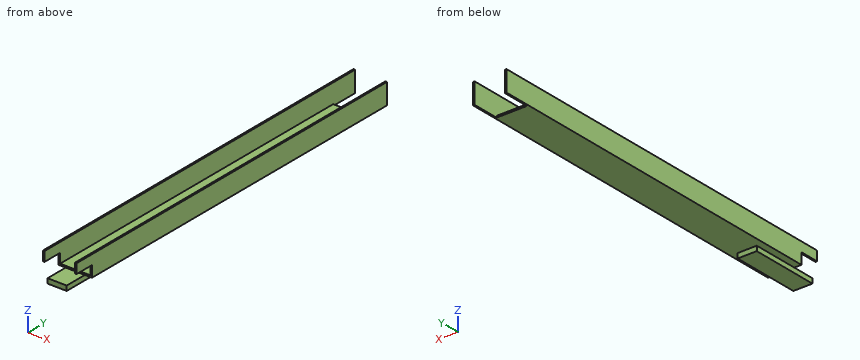
```python
from build123d import *

# Parameters (mm, degrees)
BOSS_EXTRUDE1_DEPTH = 240
SKETCH3_W           = 19
SKETCH3_H           = 1
CUT_EXTRUDE1_DEPTH  = 17
SKETCH4_W           = 19
SKETCH4_H           = 1
CUT_EXTRUDE2_DEPTH  = 11
SKETCH5_W           = 12
SKETCH5_H           = 30
BOSS_EXTRUDE2_DEPTH = 3
SKETCH6_W           = 12
SKETCH6_H           = 3
BOSS_EXTRUDE3_DEPTH = 13
SKETCH7_W           = 7
SKETCH7_H           = 12
CUT_EXTRUDE3_DEPTH  = 30


with BuildPart() as part:
    # Sketch2 → Boss-Extrude1 (new body)
    with BuildSketch(Plane(origin=(0, 0, 0), x_dir=(1, 0, 0), z_dir=(0, 1, 0))):
        Polygon((-10.5, -6.5), (-10.5, 6.5), (10.5, 6.5), (10.5, -6.5), (9.5, -6.5), (9.5, 5.5), (-9.5, 5.5), (-9.5, -6.5), align=None)
    extrude(amount=BOSS_EXTRUDE1_DEPTH)

    # Sketch3 → Cut-Extrude1 (cut)
    with BuildSketch(Plane(origin=(0, 240, 0), x_dir=(1, 0, 0), z_dir=(0, 1, 0))):
        with Locations((0, 6)):
            Rectangle(SKETCH3_W, SKETCH3_H)
    extrude(amount=-CUT_EXTRUDE1_DEPTH, mode=Mode.SUBTRACT)

    # Sketch4 → Cut-Extrude2 (cut)
    with BuildSketch(Plane.XZ):
        with Locations((0, -6)):
            Rectangle(SKETCH4_W, SKETCH4_H)
    extrude(amount=-CUT_EXTRUDE2_DEPTH, mode=Mode.SUBTRACT)

    # Sketch5 → Boss-Extrude2 (add)
    with BuildSketch(Plane(origin=(0, 0, -6.5), x_dir=(-1, 0, 0), z_dir=(0, 0, -1))):
        with Locations((0, 26)):
            Rectangle(SKETCH5_W, SKETCH5_H)
    extrude(amount=BOSS_EXTRUDE2_DEPTH)

    # Sketch6 → Boss-Extrude3 (add)
    with BuildSketch(Plane.XZ.offset(-11)):
        with Locations((0, -8)):
            Rectangle(SKETCH6_W, SKETCH6_H)
    extrude(amount=BOSS_EXTRUDE3_DEPTH)

    # Sketch7 → Cut-Extrude3 (cut)
    with BuildSketch(Plane(origin=(10.5, 0, 0), x_dir=(0, 0, -1), z_dir=(1, 0, 0))):
        with Locations((3, 6)):
            Rectangle(SKETCH7_W, SKETCH7_H)
    extrude(amount=-CUT_EXTRUDE3_DEPTH, mode=Mode.SUBTRACT)


solid = part.part
```
Can you work these out from the model? Positions are in its coordinate system, mm. Coordinates: 2 decimals unless noted, no trailing zeros. Loops run counter-clockwise (first coordinate to the right, second up) from the corner with the lowest first, then second, coordinate; pieces in that order, holes last. Notation, with made-up numbers: M 58,1 L 94,1 A17 ccw 94,20 Z; hole C -35.5,79.25 d4. An arc over 180 degrees is marked long. Put each result on its own line as item: value. Start each with the question number.
(1) Imagine slicing it at D-D on y = 103.5. List the corners of the cut face in (x, z) for me.
(2) Will these pins go through, and if not, where does the flat tip stop? pin 1 Ø0.8 at (x, y) = (-10, 7.5) entering from -Z; pin 2 Ø1 at (x, y) = (8, 188) entering from -Z; pin 3 Ø0.9 at (y, z) = (22, -7.5) entering from -X.
(3) I need wall thicknesses on probe 1 along X at (y, z) = (49, 1.75); probe 2 along Y at (x, z) = (-5.75, -6.25); probe 3 along Z at (x, y) = (-1.25, 8). Which ranges of each line are inside material? Lowest first, please.
(4) Imagine slicing it at B-B on y = 37.5. List the corners of the cut face in (x, z) for me.
(5) Imagine slicing it at A-A on z = -3.5. List the corners of the cut face in (x, y) for me, and give its area (3 significant figures).
(6) Imagine slicing it at C-C on x = -2.75. List the corners of the cut face in (y, z) for me, and give its area (3 significant figures).
Worked answers:
1. outline: M -10.5,-6.5 L 10.5,-6.5 L 10.5,6.5 L 9.5,6.5 L 9.5,-5.5 L -9.5,-5.5 L -9.5,6.5 L -10.5,6.5 Z
2. pin 1: stops at z = 0.5
2. pin 2: stops at z = -6.5
2. pin 3: stops at x = -6
3. probe 1: x = -10.5 to -9.5, 9.5 to 10.5
3. probe 2: y = 12 to 223
3. probe 3: z = -9.5 to -6.5
4. outline: M -10.5,-6.5 L -6,-6.5 L -6,-9.5 L 6,-9.5 L 6,-6.5 L 10.5,-6.5 L 10.5,6.5 L 9.5,6.5 L 9.5,-5.5 L -9.5,-5.5 L -9.5,6.5 L -10.5,6.5 Z
5. outline: M -10.5,12 L -9.5,12 L -9.5,240 L -10.5,240 Z; M 9.5,12 L 10.5,12 L 10.5,240 L 9.5,240 Z
5. area: 456 mm2
6. outline: M -2,-9.5 L 41,-9.5 L 41,-6.5 L 223,-6.5 L 223,-5.5 L 12,-5.5 L 12,-6.5 L -2,-6.5 Z
6. area: 340 mm2
